from build123d import *

# Parameters (mm, degrees)
SKETCH152_R     = 1.55
SKETCH152_R_2   = 2.05
SKETCH152_R_3   = 1.05
PAD060_DEPTH    = 4
POCKET075_DEPTH = 4.001
POCKET076_DEPTH = 4.001
FILLET004_R     = 0.8


with BuildPart() as part:
    # Sketch152 → Pad060 (new body)
    with BuildSketch(Plane.XY):
        with BuildLine():
            Line((-22, 28), (-45, 28))
            ThreePointArc((-45, 28), (-48.535534, 26.535534), (-50, 23))
            Line((-50, 23), (-50, 10.1))
            ThreePointArc((-51.5, 8.6), (-50.43934, 9.03934), (-50, 10.1))
            Line((-51.5, 8.6), (-54.8, 8.6))
            ThreePointArc((-54.8, 8.6), (-55.86066, 8.16066), (-56.3, 7.1))
            Line((-56.3, 7.1), (-56.3, -17.47))
            ThreePointArc((-56.3, -17.47), (-55.86066, -18.53066), (-54.8, -18.97))
            Line((-51.5, -18.97), (-54.8, -18.97))
            ThreePointArc((-50, -20.47), (-50.43934, -19.40934), (-51.5, -18.97))
            Line((-50, -20.47), (-50, -30))
            ThreePointArc((-50, -30), (-48.535534, -33.535534), (-45, -35))
            Line((-45, -35), (-22, -35))
            ThreePointArc((-22, -35), (-19.148569, -34.726484), (-16.401127, -33.915912))
            Line((-16.401127, -33.915912), (5.056404, -25.282774))
            ThreePointArc((5.056404, -25.282774), (6.650208, -23.995012), (7.25, -22.035728))
            Line((7.25, 22.035728), (7.25, -22.035728))
            ThreePointArc((7.25, 22.035728), (6.348838, 24.380092), (4.109405, 25.517226))
            Line((-17.892512, 27.788548), (4.109405, 25.517226))
            ThreePointArc((-17.892512, 27.788548), (-19.943537, 27.947102), (-22, 28))
        make_face()
        with Locations((0, 21.75)):
            Circle(SKETCH152_R, mode=Mode.SUBTRACT)
        with Locations((0, -21.75)):
            Circle(SKETCH152_R, mode=Mode.SUBTRACT)
        Circle(SKETCH152_R_2, mode=Mode.SUBTRACT)
        with Locations((-42.5, -30.7)):
            Circle(SKETCH152_R_2, mode=Mode.SUBTRACT)
        with Locations((-27.5, -30.7)):
            Circle(SKETCH152_R_2, mode=Mode.SUBTRACT)
        with Locations((-42.5, 23.3)):
            Circle(SKETCH152_R_2, mode=Mode.SUBTRACT)
        with Locations((-27.5, 23.3)):
            Circle(SKETCH152_R_2, mode=Mode.SUBTRACT)
        with Locations((-52.65, 5)):
            Circle(SKETCH152_R_3, mode=Mode.SUBTRACT)
        with Locations((-52.65, -15.32)):
            Circle(SKETCH152_R_3, mode=Mode.SUBTRACT)
    extrude(amount=PAD060_DEPTH)

    # Sketch153 (on Face31 of Pad060) → Pocket075 (cut, through all)
    with BuildSketch(Plane.XY.offset(4)):
        with BuildLine():
            Line((-42.5, -26.5), (-30.5, -26.5))
            ThreePointArc((-30.5, -26.5), (-29.085786, -25.914214), (-28.5, -24.5))
            Line((-28.5, -24.5), (-28.5, -15))
            ThreePointArc((-28.5, -15), (-29.085786, -13.585786), (-30.5, -13))
            Line((-30.5, -13), (-42.5, -13))
            ThreePointArc((-42.5, -13), (-43.914214, -13.585786), (-44.5, -15))
            Line((-44.5, -15), (-44.5, -24.5))
            ThreePointArc((-44.5, -24.5), (-43.914214, -25.914214), (-42.5, -26.5))
        make_face()
        with BuildLine():
            Line((-41, -7.5), (-32, -7.5))
            ThreePointArc((-32, -7.5), (-29.87868, -6.62132), (-29, -4.5))
            Line((-29, -4.5), (-29, 4.5))
            ThreePointArc((-29, 4.5), (-29.87868, 6.62132), (-32, 7.5))
            Line((-32, 7.5), (-41, 7.5))
            ThreePointArc((-41, 7.5), (-43.12132, 6.62132), (-44, 4.5))
            Line((-44, 4.5), (-44, -4.5))
            ThreePointArc((-44, -4.5), (-43.12132, -6.62132), (-41, -7.5))
        make_face()
        with BuildLine():
            Line((-40.5, 13), (-32.5, 13))
            ThreePointArc((-32.5, 13), (-31.085786, 13.585786), (-30.5, 15))
            Line((-30.5, 15), (-30.5, 18.5))
            ThreePointArc((-30.5, 18.5), (-31.085786, 19.914214), (-32.5, 20.5))
            Line((-32.5, 20.5), (-40.5, 20.5))
            ThreePointArc((-40.5, 20.5), (-41.914214, 19.914214), (-42.5, 18.5))
            Line((-42.5, 18.5), (-42.5, 15))
            ThreePointArc((-42.5, 15), (-41.914214, 13.585786), (-40.5, 13))
        make_face()
    extrude(amount=-POCKET075_DEPTH, mode=Mode.SUBTRACT)

    # Sketch154 (on Face5 of Pocket075) → Pocket076 (cut, through all)
    with BuildSketch(Plane.XY.offset(4)):
        with BuildLine():
            ThreePointArc((-4.582576, -2), (-1.119662, -4.873023), (3.25, -3.799671))
            Line((3.25, -3.799671), (3.25, -19.418155))
            ThreePointArc((3.25, -19.418155), (1.115199, -17.908603), (-1.49608, -18.040317))
            Line((-1.49608, -18.040317), (-22, -2))
            Line((-22, -2), (-4.582576, -2))
        make_face()
        with BuildLine():
            ThreePointArc((-3.957905, 22.32878), (-3.999988, 21.759892), (-3.960719, 21.190802))
            Line((-22, 7.078584), (-3.960719, 21.190802))
            Line((-22, 24), (-22, 7.078584))
            ThreePointArc((-18.303261, 23.809693), (-20.149183, 23.952392), (-22, 24))
            Line((-3.957905, 22.32878), (-18.303261, 23.809693))
        make_face()
        with BuildLine():
            Line((3.25, 19.418155), (3.25, 3.799671))
            ThreePointArc((3.25, 3.799671), (-1.119662, 4.873023), (-4.582576, 2))
            Line((-22, 2), (-4.582576, 2))
            Line((-1.49608, 18.040317), (-22, 2))
            ThreePointArc((-1.49608, 18.040317), (1.115199, 17.908603), (3.25, 19.418155))
        make_face()
        with BuildLine():
            Line((-17.89416, -30.205002), (-3.115319, -24.258942))
            ThreePointArc((-3.960719, -21.190802), (-3.856287, -22.812568), (-3.115319, -24.258942))
            Line((-3.960719, -21.190802), (-22, -7.078584))
            Line((-22, -7.078584), (-22, -31))
            ThreePointArc((-22, -31), (-19.908951, -30.799422), (-17.89416, -30.205002))
        make_face()
    extrude(amount=-POCKET076_DEPTH, mode=Mode.SUBTRACT)

    # Fillet004
    fillet004_edges = [part.edges().sort_by_distance(p)[0] for p in [
        (-22, -7.078584, 2),
        (-22, -2, 2),
        (-3.960719, -21.190802, 2),
        (-3.115319, -24.258942, 2),
        (-22, -31, 2),
        (-22, 2, 2),
        (-1.49608, 18.040317, 2),
        (3.25, 19.418155, 2),
        (-4.582576, 2, 2),
        (3.25, 3.799671, 2),
        (-22, 7.078584, 2),
        (-22, 24, 2),
        (-3.957905, 22.32878, 2),
        (-3.960719, 21.190802, 2),
        (3.25, -3.799671, 2),
        (-4.582576, -2, 2),
        (-1.49608, -18.040317, 2),
        (3.25, -19.418155, 2),
    ]]
    fillet(fillet004_edges, radius=FILLET004_R)


with BuildPart() as part_1:
    # Body022 placement: moved
    add(part.part.moved(Location((0, 0, 8.1))))


solid = part_1.part
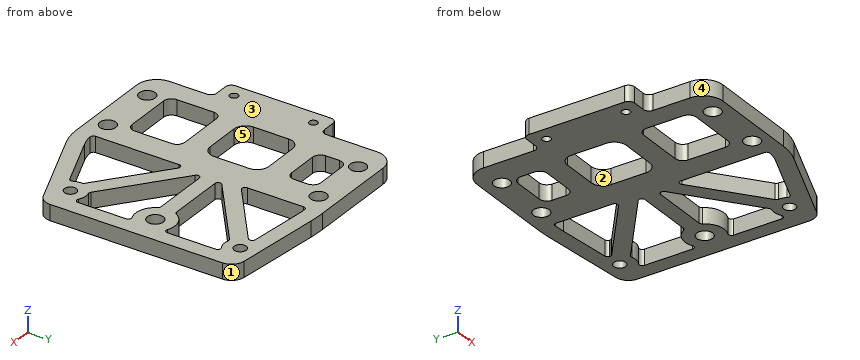
CAD build for the part. Positions are in the model's coordinates, mm. Face numbers are marked on the shaded views. A direction names the side the tool comes from. Coordinates: 2 decimals unless noted, no trailing zeros. Loops run counter-clockwise (first coordinate to the right, second up) from the corner with the lowest first, then second, coordinate; pieces in that order, holes last. Notation, with made-up numbers: (7.5, 78) - (42.5, 78) arc R3 ccw to (42.5, 83) - close; hole circle Ø1 at (-24.75, 41). An arc over 180 degrees is marked (long way). Use one line per item in the form item = value. Start each with the question number.
1) Band-saw the part on B-B (y = 0). Give the cut face in (x, z), and give its area (3 significant figures).
2) Band-saw the part on D-D (x = -14.5). Give the cut face in (y, z).
3) Band-saw the part on A-A (x = -52.65). Give the cut face in (y, z).
4) Drill centre lines: L1, parallel to Y at x = -34, z = 9.2; L2, parallel to Y at x = -27.5, z = 9.3; L3, parallel to X at y = -0.5, z = 8.7. Where is each one in solid material? Low to high. Write a range as from..to.
5) Two-plate mould, pull along Y, no slides. Class the marked faces 1, 2 and 3: +Y half, -Y half, draft (parallel to the pull), parting line (faces both ways), or undercut.
6) Tool access for the marked faces 4 and 5: list every direction of +Z, -Z, +X, -X, +Y, -Y with a clear straight run to the whole face (end or side of a thin tool).
7) Flat gauge pins, fed straight in: pin 1 (1.6 mm diameter, centred on x = -52.5, z = 10.5, fed in from +Y); pin 2 (1.2 mm diameter, centred on x = -12, z = 9.5, fed in from +Y); pin 3 (1.2 mm diameter, centred on y = 12, z = 11, fed in from -X). Where does each tip first touch, or does it go through?
8) Band-saw the part on C-C (x = 0). Give the cut face in (y, z).
Check values:
q1.outline = (-56.3, 8.1) - (-44, 8.1) - (-44, 12.1) - (-56.3, 12.1) - close; (-29, 8.1) - (-2.05, 8.1) - (-2.05, 12.1) - (-29, 12.1) - close; (2.05, 8.1) - (7.25, 8.1) - (7.25, 12.1) - (2.05, 12.1) - close
q1.area = 178 mm2
q2.outline = (-33.15, 8.1) - (-28.84, 8.1) - (-28.84, 12.1) - (-33.15, 12.1) - close; (-12.95, 8.1) - (-7.87, 8.1) - (-7.87, 12.1) - (-12.95, 12.1) - close; (-2, 8.1) - (2, 8.1) - (2, 12.1) - (-2, 12.1) - close; (7.87, 8.1) - (12.95, 8.1) - (12.95, 12.1) - (7.87, 12.1) - close; (23.42, 8.1) - (27.44, 8.1) - (27.44, 12.1) - (23.42, 12.1) - close
q3.outline = (-18.97, 8.1) - (-16.37, 8.1) - (-16.37, 12.1) - (-18.97, 12.1) - close; (-14.27, 8.1) - (3.95, 8.1) - (3.95, 12.1) - (-14.27, 12.1) - close; (6.05, 8.1) - (8.6, 8.1) - (8.6, 12.1) - (6.05, 12.1) - close
q4.L1 = -35..-26.5, -13..-7.5, 7.5..13, 20.5..28
q4.L2 = -35..-32.75, -28.65..21.25, 25.35..28
q4.L3 = -56.3..-44, -29..-1.99, 1.99..7.25
q5.face_1 = +Y half
q5.face_2 = undercut
q5.face_3 = draft
q6.face_4 = +Z, -Z, -X, -Y
q6.face_5 = +Z, -Z
q7.pin_1 = 8.6
q7.pin_2 = 27.24
q7.pin_3 = -50
q8.outline = (-27.32, 8.1) - (-23.3, 8.1) - (-23.3, 12.1) - (-27.32, 12.1) - close; (-20.2, 8.1) - (-17.75, 8.1) - (-17.75, 12.1) - (-20.2, 12.1) - close; (-5, 8.1) - (-2.05, 8.1) - (-2.05, 12.1) - (-5, 12.1) - close; (2.05, 8.1) - (5, 8.1) - (5, 12.1) - (2.05, 12.1) - close; (17.75, 8.1) - (20.2, 8.1) - (20.2, 12.1) - (17.75, 12.1) - close; (23.3, 8.1) - (25.94, 8.1) - (25.94, 12.1) - (23.3, 12.1) - close
